from build123d import *

# Parameters (mm, degrees)
SKETCH1_W           = 40
SKETCH1_H           = 96.5
BOSS_EXTRUDE1_DEPTH = 4
CUT_EXTRUDE3_DEPTH  = 20
SKETCH5_R           = 2
CUT_EXTRUDE5_DEPTH  = 10
SKETCH6_W           = 2
SKETCH6_H           = 96.5
CUT_EXTRUDE6_DEPTH  = 10
SKETCH7_W           = 36
SKETCH7_H           = 96.5
SKETCH7_R           = 2
BOSS_EXTRUDE2_DEPTH = 2
CUT_EXTRUDE7_DEPTH  = 97.5
SKETCH8_R           = 4.25
SKETCH8_R_2         = 2
CUT_EXTRUDE8_DEPTH  = 3.5
CUT_EXTRUDE10_DEPTH = 122
SKETCH10_W          = 36
SKETCH10_H          = 6
BOSS_EXTRUDE3_DEPTH = 2


with BuildPart() as part:
    # Sketch1 → Boss-Extrude1 (new body)
    with BuildSketch(Plane.XY):
        with Locations((0.330243162, -38.25)):
            Rectangle(SKETCH1_W, SKETCH1_H)
    extrude(amount=BOSS_EXTRUDE1_DEPTH)

    # Sketch3 → Cut-Extrude3 (cut)
    with BuildSketch(Plane.XZ.offset(86.5)):
        Polygon((-12.106417754, 4), (-10.650536835, 0), (-7.858578609, 0), (-11.858578609, 4), align=None)
        Polygon((11.858580346, 4), (7.858579777, 0), (10.650537342, 0), (12.106418599, 4), align=None)
    extrude(amount=-CUT_EXTRUDE3_DEPTH, mode=Mode.SUBTRACT)

    # Sketch5 → Cut-Extrude5 (cut)
    with BuildSketch(Plane.XY.offset(4)):
        Circle(SKETCH5_R)
        with Locations((0, -76.5)):
            Circle(SKETCH5_R)
    extrude(amount=-CUT_EXTRUDE5_DEPTH, mode=Mode.SUBTRACT)

    # Sketch6 → Cut-Extrude6 (cut)
    with BuildSketch(Plane.XY.offset(4)):
        with Locations((-18.669756838, -38.25)):
            Rectangle(SKETCH6_W, SKETCH6_H)
        with Locations((19.330243162, -38.25)):
            Rectangle(SKETCH6_W, SKETCH6_H)
    extrude(amount=-CUT_EXTRUDE6_DEPTH, mode=Mode.SUBTRACT)

    # Sketch7 → Boss-Extrude2 (add)
    with BuildSketch(Plane.XY.offset(4)):
        with Locations((0.330243162, -38.25)):
            Rectangle(SKETCH7_W, SKETCH7_H)
        with Locations((0, -76.5)):
            Circle(SKETCH7_R, mode=Mode.SUBTRACT)
        Circle(SKETCH7_R, mode=Mode.SUBTRACT)
    extrude(amount=BOSS_EXTRUDE2_DEPTH)

    # Sketch4 → Cut-Extrude7 (cut, through all)
    with BuildSketch(Plane(origin=(0, 10, 0), x_dir=(1, 0, 0), z_dir=(0, 1, 0))):
        Polygon((-11.858578609, -4), (-7.858578609, 0), (-10.650536835, 0), (-12.106417754, -4), align=None)
        Polygon((10.650537342, 0), (7.858579777, 0), (11.858580346, -4), (12.106418599, -4), align=None)
    extrude(amount=-CUT_EXTRUDE7_DEPTH, mode=Mode.SUBTRACT)

    # Sketch8 → Cut-Extrude8 (cut)
    with BuildSketch(Plane(origin=(0, 0, 0), x_dir=(-1, 0, 0), z_dir=(0, 0, -1))):
        Circle(SKETCH8_R)
        Circle(SKETCH8_R_2, mode=Mode.SUBTRACT)
        with Locations((0, -76.5)):
            Circle(SKETCH8_R)
        with Locations((0, -76.5)):
            Circle(SKETCH8_R_2, mode=Mode.SUBTRACT)
    extrude(amount=-CUT_EXTRUDE8_DEPTH, mode=Mode.SUBTRACT)

    # Sketch9 → Cut-Extrude10 (cut)
    with BuildSketch(Plane(origin=(0, 10, 0), x_dir=(1, 0, 0), z_dir=(0, 1, 0))):
        Polygon((-10.790578344, 0.2), (-7.375735897, 0.2), (-11.775735897, -4.2), (-12.392047354, -4.2), align=None)
        Polygon((7.375737016, 0.2), (10.790578839, 0.2), (12.392048222, -4.2), (11.775737642, -4.2), align=None)
    extrude(amount=-CUT_EXTRUDE10_DEPTH, mode=Mode.SUBTRACT)

    # Sketch10 → Boss-Extrude3 (add)
    with BuildSketch(Plane(origin=(0, 10, 0), x_dir=(1, 0, 0), z_dir=(0, 1, 0))):
        with Locations((0.330243162, -3)):
            Rectangle(SKETCH10_W, SKETCH10_H)
    extrude(amount=BOSS_EXTRUDE3_DEPTH)


solid = part.part
Verification items for the finished model (mm, model axes). A direction names the side the tool comes from. Coordinates: 2 decimals unless noted, no trailing zeros. Write each loop counter-clockwise with the first axis right and the second up, starting at its lowest first coordinate (ties: lowest second). Pieces come first, ordered by that corner, then holes. Notation, with made-up numbers: M -28.5,6 L 8.5,6 A18 cw 8.5,29 Z; hole C 35,19.25 d2. An arc over 180 degrees is marked long. One line per question, with ' | ' between items.
1) Release check for a two-part mould opening along Y. For faces 1 (the face through (11.617, -37.574, 2.071)), 2 (the face through (10, 10, 2)), 3 (the face through (0, -2, 5)) record: +Y half, -Y half, draft (parallel to the pull), parting line (faces both ways), or undercut.
Solutions:
face 1: draft | face 2: -Y half | face 3: undercut
2) Sectioned sample at A-A on x = 0. Record the cut outline in (y, z), then the cut area to 4 significant figures.
Solutions:
outline: M -86.5,0 L -80.75,0 L -80.75,3.5 L -78.5,3.5 L -78.5,6 L -86.5,6 Z; M -74.5,3.5 L -72.25,3.5 L -72.25,0 L -4.25,0 L -4.25,3.5 L -2,3.5 L -2,6 L -74.5,6 Z; M 2,3.5 L 4.25,3.5 L 4.25,0 L 12,0 L 12,6 L 2,6 Z | area: 511.5 mm^2
3) Sectioned sample at B-B on y = -76.5. Record the cut outline in (x, z).
Solutions:
outline: M -17.67,0 L -10.86,0 L -12.39,4.2 L -11.78,4.2 L -7.58,0 L -4.25,0 L -4.25,3.5 L -2,3.5 L -2,6 L -17.67,6 Z; M 2,3.5 L 4.25,3.5 L 4.25,0 L 7.58,0 L 11.78,4.2 L 12.39,4.2 L 10.86,0 L 18.33,0 L 18.33,6 L 2,6 Z
4) Sectioned sample at C-C on z = 1.75. Record the cut outline in (x, y), then the cut area to 3 significant figures.
Solutions:
outline: M -17.67,-86.5 L -11.5,-86.5 L -11.5,10 L -9.33,10 L -9.33,-86.5 L 9.33,-86.5 L 9.33,10 L 11.5,10 L 11.5,-86.5 L 18.33,-86.5 L 18.33,12 L -17.67,12 Z; hole C 0,-76.5 d8.5; hole C 0,0 d8.5 | area: 3,010 mm^2
5) Material ranges on L1, parallel to Y at x = 0, z = 1; L2, parallel to Y at x = 0, z = 5.35; L3, parallel to X at y = -76.5, z = 4.45, recorded low to high.
Solutions:
L1: -86.5 to -80.75, -72.25 to -4.25, 4.25 to 12 | L2: -86.5 to -78.5, -74.5 to -2, 2 to 12 | L3: -17.67 to -2, 2 to 18.33
6) Depth check by flat-ended pin: pin 1 Ø3 at (x, y) = (0, 0) entering from -Z; pin 2 Ø4 at (x, y) = (1, 0) entering from -Z. Enter the tip coordinate at first touch or a pass-through.
Solutions:
pin 1: through | pin 2: z = 3.5
7) Access from +Z, -Z, +X, -X, +Y, -Y to the whole of each face (thin tool, end or side, straight path). Record for faces 4 (the face through (-11.64, -37.57, 2.13)), 5 (the face through (0, -38, 0)), 6 (the face through (-2.285, 3.584, 1.726)).
Solutions:
face 4: -Y | face 5: -Z, +X, -X, +Y, -Y | face 6: -Z
